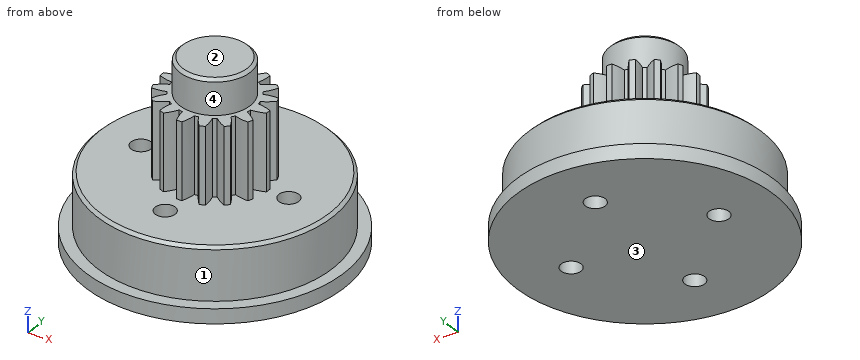
Autodesk Inventor part; units mm, degrees
ref_plane "YZ Plane" through (0, 0, 0) normal (1, 0, 0) x (0, 1, 0)
ref_plane "XZ Plane" through (0, 0, 0) normal (0, 1, 0) x (-1, 0, 0)
ref_plane "XY Plane" through (0, 0, 0) normal (0, 0, 1) x (1, 0, 0)
sketch "スケッチ1" plane through (0, 0, 0) normal (1, 0, 0) x (0, 1, 0)
  line L0 (22, 0) -> (22, 2.5)
  line L1 (22, 2.5) -> (20, 2.5)
  line L2 (20, 2.5) -> (20, 11.5)
  line L3 (20, 11.5) -> (0, 11.5)
  line L4 (0, 11.5) -> (0, 0)
  line L5 (0, 0) -> (22, 0)
  dimension "d0" = 20
  dimension "d1" = 9
  dimension "d2" = 2.5
  dimension "d3" = 2
revolve "回転1" add sketch "スケッチ1" angle 360 about axis through (0, 0, 11.5) along (0, 0, -1)
sketch "スケッチ2" plane through (0, 0, 11.5) normal (0, 0, 1) x (1, 0, 0)
  arc A0 (-3.8476, 8.135) -> (-3.4702, 5.7897) centre (3.494, 8.1133) ccw
  arc A1 (-3.4702, 5.7897) -> (-4.021, 5.4217) centre (0, 0) ccw
  arc A2 (-4.021, 5.4217) -> (-6.0434, 6.6678) centre (-8.8328, -0.1232) ccw
  arc A3 (-6.0434, 6.6678) -> (-6.6678, 6.0434) centre (0, 0) ccw
  arc A4 (-6.6678, 6.0434) -> (-5.4217, 4.021) centre (0.1232, 8.8328) ccw
  arc A5 (-5.4217, 4.021) -> (-5.7897, 3.4702) centre (0, 0) ccw
  arc A6 (-5.7897, 3.4702) -> (-8.135, 3.8476) centre (-8.1133, -3.494) ccw
  arc A7 (-8.135, 3.8476) -> (-8.473, 3.0317) centre (0, 0) ccw
  arc A8 (-8.473, 3.0317) -> (-6.5477, 1.6401) centre (-3.2664, 8.2076) ccw
  arc A9 (-6.5477, 1.6401) -> (-6.6769, 0.9904) centre (0, 0) ccw
  arc A10 (-6.6769, 0.9904) -> (-8.9882, 0.4416) centre (-6.1586, -6.3328) ccw
  arc A11 (-8.9882, 0.4416) -> (-8.9882, -0.4416) centre (0, 0) ccw
  arc A12 (-8.9882, -0.4416) -> (-6.6769, -0.9904) centre (-6.1586, 6.3328) ccw
  arc A13 (-6.6769, -0.9904) -> (-6.5477, -1.6401) centre (0, 0) ccw
  arc A14 (-6.5477, -1.6401) -> (-8.473, -3.0317) centre (-3.2664, -8.2076) ccw
  arc A15 (-8.473, -3.0317) -> (-8.135, -3.8476) centre (0, 0) ccw
  arc A16 (-8.135, -3.8476) -> (-5.7897, -3.4702) centre (-8.1133, 3.494) ccw
  arc A17 (-5.7897, -3.4702) -> (-5.4217, -4.021) centre (0, 0) ccw
  arc A18 (-5.4217, -4.021) -> (-6.6678, -6.0434) centre (0.1232, -8.8328) ccw
  arc A19 (-6.6678, -6.0434) -> (-6.0434, -6.6678) centre (0, 0) ccw
  arc A20 (-6.0434, -6.6678) -> (-4.021, -5.4217) centre (-8.8328, 0.1232) ccw
  arc A21 (-4.021, -5.4217) -> (-3.4702, -5.7897) centre (0, 0) ccw
  arc A22 (-3.4702, -5.7897) -> (-3.8476, -8.135) centre (3.494, -8.1133) ccw
  arc A23 (-3.8476, -8.135) -> (-3.0317, -8.473) centre (0, 0) ccw
  arc A24 (-3.0317, -8.473) -> (-1.6401, -6.5477) centre (-8.2076, -3.2664) ccw
  arc A25 (-1.6401, -6.5477) -> (-0.9904, -6.6769) centre (0, 0) ccw
  arc A26 (-0.9904, -6.6769) -> (-0.4416, -8.9882) centre (6.3328, -6.1586) ccw
  arc A27 (-0.4416, -8.9882) -> (0.4416, -8.9882) centre (0, 0) ccw
  arc A28 (0.4416, -8.9882) -> (0.9904, -6.6769) centre (-6.3328, -6.1586) ccw
  arc A29 (0.9904, -6.6769) -> (1.6401, -6.5477) centre (0, 0) ccw
  arc A30 (1.6401, -6.5477) -> (3.0317, -8.473) centre (8.2076, -3.2664) ccw
  arc A31 (3.0317, -8.473) -> (3.8476, -8.135) centre (0, 0) ccw
  arc A32 (3.8476, -8.135) -> (3.4702, -5.7897) centre (-3.494, -8.1133) ccw
  arc A33 (3.4702, -5.7897) -> (4.021, -5.4217) centre (0, 0) ccw
  arc A34 (4.021, -5.4217) -> (6.0434, -6.6678) centre (8.8328, 0.1232) ccw
  arc A35 (6.0434, -6.6678) -> (6.6678, -6.0434) centre (0, 0) ccw
  arc A36 (6.6678, -6.0434) -> (5.4217, -4.021) centre (-0.1232, -8.8328) ccw
  arc A37 (5.4217, -4.021) -> (5.7897, -3.4702) centre (0, 0) ccw
  arc A38 (5.7897, -3.4702) -> (8.135, -3.8476) centre (8.1133, 3.494) ccw
  arc A39 (8.135, -3.8476) -> (8.473, -3.0317) centre (0, 0) ccw
  arc A40 (8.473, -3.0317) -> (6.5477, -1.6401) centre (3.2664, -8.2076) ccw
  arc A41 (6.5477, -1.6401) -> (6.6769, -0.9904) centre (0, 0) ccw
  arc A42 (6.6769, -0.9904) -> (8.9882, -0.4416) centre (6.1586, 6.3328) ccw
  arc A43 (8.9882, -0.4416) -> (8.9882, 0.4416) centre (0, 0) ccw
  arc A44 (8.9882, 0.4416) -> (6.6769, 0.9904) centre (6.1586, -6.3328) ccw
  arc A45 (6.6769, 0.9904) -> (6.5477, 1.6401) centre (0, 0) ccw
  arc A46 (6.5477, 1.6401) -> (8.473, 3.0317) centre (3.2664, 8.2076) ccw
  arc A47 (8.473, 3.0317) -> (8.135, 3.8476) centre (0, 0) ccw
  arc A48 (8.135, 3.8476) -> (5.7897, 3.4702) centre (8.1133, -3.494) ccw
  arc A49 (5.7897, 3.4702) -> (5.4217, 4.021) centre (0, 0) ccw
  arc A50 (5.4217, 4.021) -> (6.6678, 6.0434) centre (-0.1232, 8.8328) ccw
  arc A51 (6.6678, 6.0434) -> (6.0434, 6.6678) centre (0, 0) ccw
  arc A52 (6.0434, 6.6678) -> (4.021, 5.4217) centre (8.8328, -0.1232) ccw
  arc A53 (4.021, 5.4217) -> (3.4702, 5.7897) centre (0, 0) ccw
  arc A54 (3.4702, 5.7897) -> (3.8476, 8.135) centre (-3.494, 8.1133) ccw
  arc A55 (3.8476, 8.135) -> (3.0317, 8.473) centre (0, 0) ccw
  arc A56 (3.0317, 8.473) -> (1.6401, 6.5477) centre (8.2076, 3.2664) ccw
  arc A57 (1.6401, 6.5477) -> (0.9904, 6.6769) centre (0, 0) ccw
  arc A58 (0.9904, 6.6769) -> (0.4416, 8.9882) centre (-6.3328, 6.1586) ccw
  arc A59 (0.4416, 8.9882) -> (-0.4416, 8.9882) centre (0, 0) ccw
  arc A60 (-0.4416, 8.9882) -> (-0.9904, 6.6769) centre (6.3328, 6.1586) ccw
  arc A61 (-0.9904, 6.6769) -> (-1.6401, 6.5477) centre (0, 0) ccw
  arc A62 (-1.6401, 6.5477) -> (-3.0317, 8.473) centre (-8.2076, 3.2664) ccw
  arc A63 (-3.0317, 8.473) -> (-3.8476, 8.135) centre (0, 0) ccw
  point P0 (0, 0)
extrude "押し出し1" add sketch "スケッチ2" along normal blind 13
sketch "スケッチ3" plane through (0, 0, 24.5) normal (0, 0, 1) x (1, 0, 0)
  circle A0 centre (0, 0) radius 6
  dimension "d7" = 12
extrude "押し出し2" add sketch "スケッチ3" along normal blind 6
chamfer "面取り1" distance 0.5 angle 45 2 edges at (-6, 0, 30.5) (0, -20, 11.5)
sketch "スケッチ4" plane through (0, 0, 11.5) normal (0, 0, 1) x (1, 0, 0)
  circle A0 centre (0, 0) radius 12.5
  point P0 (0, 0)
  point P1 (0, 12.5)
  point P2 (-12.5, 0)
  point P3 (0, -12.5)
  point P4 (12.5, 0)
  dimension "d13" = 25
  dimension "d16" = 360
hole "穴1" at (0, 12.5, 11.5) at (-12.5, 0, 11.5) at (0, -12.5, 11.5) at (12.5, 0, 11.5) direction (0, 0, -1) diameter 3.4 end through all
properties part number "s-assy-sun_gear" material "ABS プラスチック"
Geometry: final body of the model. Coordinates: model frame, mm. Face numbers are marked on the shaded views. A direction names the side the tool comes from. Give positions to 0.01 mm unless a question says otherwise; leave off trailing zeros. Loops run counter-clockwise (first coordinate to the right, second up) from the corner with the lowest first, then second, coordinate; pieces in that order, holes last. Notation, with made-up numbers: M 32,7.5 L 64,7.5 A23 cw 64,25.5 Z; hole C 89.5,27.5 d8. An arc over 180 degrees is marked long. Put each result on its own line as item: value. Start each with the question number.
1) Access query for the marked faces 3 and 4. Directions: +Z, -Z, +X, -X, +Y, -Y. A direction counts if a zero-diameter tool reaches every point of the face in a straight line with its end or side. Return the directions, or none.
2) Pull-direction query (X, two-part tool) for the marked faces 1 and 2; classes: pulls with the +X half, pulls with the -X half, needs draft (parallel to the pull), parting line crosses it, or undercut.
3) Contact query for flat-ended pins moving along their axis: pin 1 (19.5 mm diameter, centred on x = -5.5, y = -1, fed in from +Z); pin 2 (2 mm diameter, centred on y = -15, z = 8.5, fed in from -X); pin 3 (3 mm diameter, centred on y = 3, z = 5.5, fed in from +X); pin 4 (2.5 mm diameter, centred on x = 12.5, y = 0, fed in from +Z). Output: stop coordinate, or through.
4) Cut plane B-B (z = 27.5). Output: boundary loops of the cut face in (x, y), then the cut area to 3 significant figures.
5) Cut plane A-A (z = 10). Output: boundary loops of the cut face in (x, y), then the cut area to 3 significant figures.
6) Ray query, line 1 along X through (y, z) = (0, 9); line 2 along Y through (x, z) = (7, 13); line 3 along Z through (x, y) = (19.5, 0). Return the intervals inside material, ascending.
Verdict:
1. face 3: -Z, +X, -X, +Y, -Y
1. face 4: +Z
2. face 1: parting line crosses it
2. face 2: needs draft
3. pin 1: z = 30.5
3. pin 2: x = -14.28
3. pin 3: x = 19.94
3. pin 4: through
4. outline: C 0,0 d12
4. area: 113 mm2
5. outline: C 0,0 d40; hole C -12.5,0 d3.4; hole C 0,-12.5 d3.4; hole C 0,12.5 d3.4; hole C 12.5,0 d3.4
5. area: 1,220 mm2
6. line 1: -20 to -14.2, -10.8 to 10.8, 14.2 to 20
6. line 2: -3.76 to -1.89, -0.96 to 0.96, 1.89 to 3.76
6. line 3: 0 to 11.5
